```python
from build123d import *

# Parameters (mm, degrees)
EXTRUDE_1_DEPTH     = 20
SKETCH_2_R          = 7
CUT_EXTRUDE_1_DEPTH = 83.097503007


with BuildPart() as part:
    # ｽｹｯﾁ1 → ﾎﾞｽ - 押し出し1 (new, symmetric)
    with BuildSketch(Plane.XY):
        with BuildLine():
            Line((73, 0), (78, 0))
            Line((78, 0), (78, 16))
            Line((78, 16), (28, 16))
            Line((28, 16), (28, 10.205732014))
            Line((28, 10.205732014), (47.449902109, 5.715368296))
            ThreePointArc((47.449902109, 5.715368296), (48.565216314, 5.01165744), (49, 3.766628167))
            Line((49, 3.766628167), (49, 3))
            Line((49, 3), (70, 3))
            ThreePointArc((70, 3), (72.121320344, 2.121320344), (73, 0))
        make_face()
    extrude(amount=EXTRUDE_1_DEPTH, both=True)

    # ｽｹｯﾁ2 → ｶｯﾄ - 押し出し1 (cut, through all)
    with BuildSketch(Plane(origin=(0, 16, 0), x_dir=(1, 0, 0), z_dir=(0, 1, 0))):
        with Locations(Location((61, 0, 0), (0, 0, 180))):
            Circle(SKETCH_2_R)
    extrude(amount=-CUT_EXTRUDE_1_DEPTH, mode=Mode.SUBTRACT)


solid = part.part
```
Model file for the job. Use its own axes, mm. Round coordinates to 2 decimals unless told otherwise and drop trailing zeros. Write each loop counter-clockwise with the first axis right and the second up, starting at its lowest first coordinate (ties: lowest second). Pieces come first, ordered by that corner, then holes. Notation, with made-up numbers: (25.5, -21.75) - (38.5, -21.75) arc R21 cw to (38.5, -1.75) - close; hole circle Ø2 at (4, 52). An arc over 180 degrees is marked (long way). One line per item, written item: value.
(1) Cut at B-B, the plane x = 61. Give the cut face in (y, z).
Values follow:
outline: (3, -20) - (16, -20) - (16, -7) - (3, -7) - close; (3, 7) - (16, 7) - (16, 20) - (3, 20) - close
(2) Two-plate mould, pull along Z, no slides. Class faces 1 (the flat face through (58, 10, 20)), 2 (the flat face through (58, 10, -20)), 3 (the flat face through (55, 3, 5)), 4 (the cylindrical face through (54.323, 9.591, 2.103)): pulls with the +Z half, pulls with the -Z half, needs draft (parallel to the pull), parting line crosses it, or undercut.
Values follow:
face 1: pulls with the +Z half
face 2: pulls with the -Z half
face 3: needs draft
face 4: undercut
(3) Cut at C-C, the plane y = 13.75. Give the cut face in (x, z), plus the area to 3 significant figures.
Values follow:
outline: (28, -20) - (78, -20) - (78, 20) - (28, 20) - close; hole circle Ø14 at (61, 0)
area: 1,850 mm²
(4) Cut at A-A, the plane z = 0. Give the cut face in (x, y), plus the area to 3 significant figures.
Values follow:
outline: (28, 10.21) - (47.45, 5.72) arc R2 cw to (49, 3.77) - (49, 3) - (54, 3) - (54, 16) - (28, 16) - close; (68, 3) - (70, 3) arc R3 cw to (73, 0) - (78, 0) - (78, 16) - (68, 16) - close
area: 385 mm²
(5) Cut at D-D, the plane z = -11. Give the cut face in (x, y).
Values follow:
outline: (28, 10.21) - (47.45, 5.72) arc R2 cw to (49, 3.77) - (49, 3) - (70, 3) arc R3 cw to (73, 0) - (78, 0) - (78, 16) - (28, 16) - close
(6) Wall check: probe 1 along Z at (x, y) = (61, 8.25); probe 2 along Y at (x, z) = (53, 15); probe 3 along X at (y, z) = (12.5, -1.5). Give the ranges that are in metal, low to high.
Values follow:
probe 1: z = -20 to -7, 7 to 20
probe 2: y = 3 to 16
probe 3: x = 28 to 54.16, 67.84 to 78
(7) Drop flat-ended pins along their axis: P1, Ø22.5, axis at x = 61, z = 0, coming from the -Y side; P2, Ø6, axis at x = 41.5, z = -14, coming from the -Y side; P3, Ø17, axis at x = 56, z = -7.5, coming from the -Y side. Give the stop position or say it passes through.
Values follow:
P1: stops at y = 1.98
P2: stops at y = 6.4
P3: stops at y = 3
